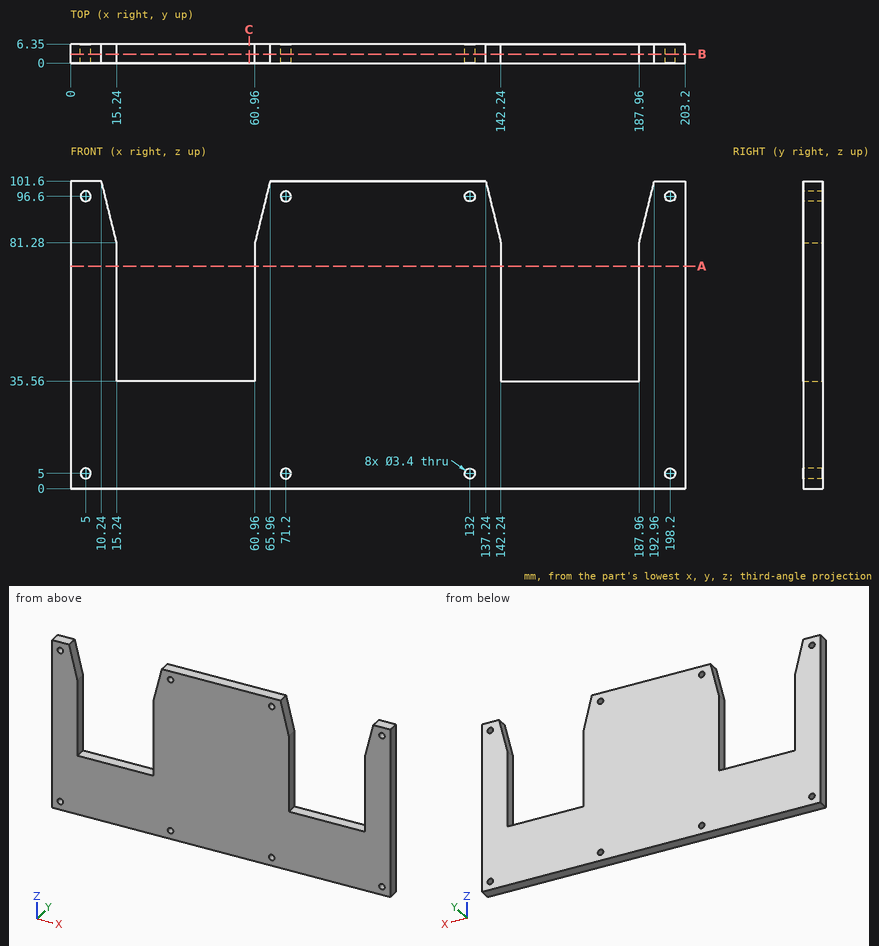
Answer from the drawing. Dimensions are ordinates in mm from the lowest x, y and z of the part. Give positions to 0.01 mm unless a question says otherwise; leave off trailing zeros. Order: outer loops, then holes, each group sorted by start corner. A loop starts at its lowest first (then second) coordinate and runs counter-clockwise, first axis right, second up.
(1) Straight lines are drawn through the part: L1, parallel to X at y = 2.5, z = 64; L2, parallel to Z at x = 198.2, y = 5; L3, parallel to X at y = 5, z = 5. For each, find the intervals that lie inside material, in ascending order.
(2) Find section B-B (y = 3). Give the number of separate pieces and of enclosed holes in the cut face, plus the area to 3 significant figures.
(3) Find section C-C (x = 59). Give the vertices of the cut face in (y, z), plus the area to 3 significant figures.
(4) Find section A-A (z = 73.5). Give the vertices of the cut face in (x, y).
(5) Given pin 1 (1.9 mm diameter, centred on y = 3, z = 53, fed in from -X), flat-ended and moving along its own axis, determine where the tip first touches the part or whether it passes through.
Result sheet:
1. L1: x = 0 to 15.24, 60.96 to 142.24, 187.96 to 203.2
1. L2: z = 0 to 3.3, 6.7 to 94.9, 98.3 to 101.6
1. L3: x = 0 to 3.3, 6.7 to 69.5, 72.9 to 130.3, 133.7 to 196.5, 199.9 to 203.2
2. separate pieces: 1
2. enclosed holes: 8
2. area: 14,300 mm2
3. outline: (0, 0) - (6.35, 0) - (6.35, 35.56) - (0, 35.56) - close
3. area: 226 mm2
4. outline: (0, 0) - (15.24, 0) - (15.24, 6.35) - (0, 6.35) - close; (60.96, 0) - (142.24, 0) - (142.24, 6.35) - (60.96, 6.35) - close; (187.96, 0) - (203.2, 0) - (203.2, 6.35) - (187.96, 6.35) - close
5. pin 1: stops at x = 0
